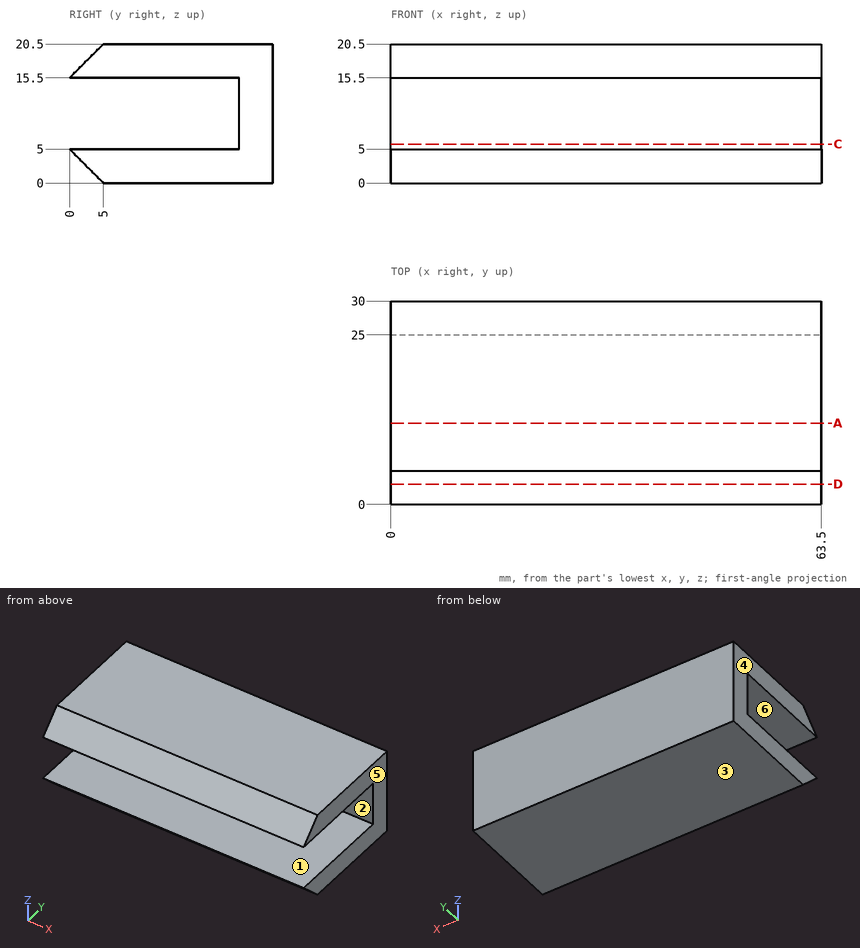
Answer from the drawing. Dimensions are ordinates in mm from the lowest x, y and z of the part. A direction names the side the tool comes from. Coordinates: 2 decimals unless noted, no trailing zeros. Loops run counter-clockwise (first coordinate to the right, second up) from the corner with the lowest first, then second, coordinate; pieces in that order, holes last. Notation, with made-up numbers: (-8, 12) - (11, 12) arc R26 cw to (11, 37) - close; hole circle Ø11 at (36, 19.5). An arc over 180 degrees is marked (long way). Answer in a Markdown table with one row per item.
1. Find section A-A, the plane y = 12. Write down the section's boundary in (x, z), then the cut area to 3 significant figures.
Conclusion:
| item | result |
|---|---|
| outline | (0, 0) - (63.5, 0) - (63.5, 5) - (0, 5) - close; (0, 15.5) - (63.5, 15.5) - (63.5, 20.5) - (0, 20.5) - close |
| area | 635 mm² |
2. Given pin 1 (5 mm diameter, centred on x = 23.5, z = 8.5, fed in from -Y), flat-ended and moving along its own axis, determine where the tip first touches the part or whether it passes through.
Conclusion:
| item | result |
|---|---|
| pin 1 | stops at y = 25 |
3. Find section C-C, the plane z = 5.75. Write down the section's boundary in (x, y).
Conclusion:
| item | result |
|---|---|
| outline | (0, 25) - (63.5, 25) - (63.5, 30) - (0, 30) - close |
4. Find section D-D, the plane y = 3. Write down the section's boundary in (x, z).
Conclusion:
| item | result |
|---|---|
| outline | (0, 2) - (63.5, 2) - (63.5, 5) - (0, 5) - close; (0, 15.5) - (63.5, 15.5) - (63.5, 18.5) - (0, 18.5) - close |
5. Determine the mould class of the marked faces 1, 2, 3 and 4 for opening direction Z: +Z half, -Z half, draft (parallel to the pull), parting line (faces both ways), or undercut.
Conclusion:
| item | result |
|---|---|
| face 1 | undercut |
| face 2 | undercut |
| face 3 | -Z half |
| face 4 | draft |
6. Which of the six approach directions +Z, -Z, +X, -X, +Y, -Y give full straight-line access (tool end or side, diameter ignored) to the marked faces 5 and 6?
Conclusion:
| item | result |
|---|---|
| face 5 | +Z, -Z, +X, +Y, -Y |
| face 6 | +X, -X, -Y |
7. Straight lines are drawn through the part: line 1 (Z direction, x = 35.5, y = 11.5); line 2 (Z direction, x = 45.5, y = 3); line 3 (Y direction, x = 9, z = 14.25). For each, find the intervals that lie inside material, in ascending order.
Conclusion:
| item | result |
|---|---|
| line 1 | z = 0 to 5, 15.5 to 20.5 |
| line 2 | z = 2 to 5, 15.5 to 18.5 |
| line 3 | y = 25 to 30 |
